from build123d import *

# Parameters (mm, degrees)
EXTRUDE_1_DEPTH              = 27
CUT_EXTRUDE_1_REACH          = 33.032
HOLE_WIZARD_M2_1_D           = 2.3
HOLE_WIZARD_M2_1_CBORE_D     = 3.8
HOLE_WIZARD_M2_1_CBORE_DEPTH = 0.5
PATTERN_LINEAR_1_COUNT       = 3
PATTERN_LINEAR_1_PITCH       = 10.5
MIRROR_1_COPY_1_D            = 2.3
MIRROR_1_COPY_1_CBORE_D      = 3.8
MIRROR_1_COPY_1_CBORE_DEPTH  = 0.5
MIRROR_1_COPY_2_D            = 2.3
MIRROR_1_COPY_2_CBORE_D      = 3.8
MIRROR_1_COPY_2_CBORE_DEPTH  = 0.5
CHAMFER_1_SIZE               = 1
MIRROR_3_COPY_1_D            = 2.3
MIRROR_3_COPY_1_CBORE_D      = 3.8
MIRROR_3_COPY_1_CBORE_DEPTH  = 0.5
MIRROR_3_COPY_2_D            = 2.3
MIRROR_3_COPY_2_CBORE_D      = 3.8
MIRROR_3_COPY_2_CBORE_DEPTH  = 0.5
MIRROR_3_COPY_3_D            = 2.3
MIRROR_3_COPY_3_CBORE_D      = 3.8
MIRROR_3_COPY_3_CBORE_DEPTH  = 0.5
MIRROR_3_COPY_4_D            = 2.3
MIRROR_3_COPY_4_CBORE_D      = 3.8
MIRROR_3_COPY_4_CBORE_DEPTH  = 0.5
MIRROR_3_COPY_5_D            = 2.3
MIRROR_3_COPY_5_CBORE_D      = 3.8
MIRROR_3_COPY_5_CBORE_DEPTH  = 0.5
CHAMFER_1_OF_MIRROR_3_SIZE   = 1
FILLET_1_R                   = 1.5
FILLET_2_R                   = 1
CHAMFER_2_SIZE               = 1.5
CUT_EXTRUDE_2_DEPTH          = 41.669398815


with BuildPart() as part:
    # ｽｹｯﾁ1 → ﾎﾞｽ - 押し出し1 (new, symmetric)
    with BuildSketch(Plane(origin=(0, 0, 0), x_dir=(0, 0, -1), z_dir=(1, 0, 0))):
        Polygon((-15, 0), (15, 0), (15, 5), (13, 5), (13, 2), (-13, 2), (-13, 5), (-15, 5), align=None)
    extrude(amount=EXTRUDE_1_DEPTH, both=True)

    # ｽｹｯﾁ2 → ｶｯﾄ - 押し出し1 (cut, up to next)
    with BuildSketch(Plane(origin=(0, 2, 0), x_dir=(1, 0, 0), z_dir=(0, 1, 0)), mode=Mode.PRIVATE) as cut_extrude_1_sk1:
        with BuildLine():
            Line((24, 6.75), (28, 6.75))
            Line((28, 6.75), (28, -6.75))
            Line((28, -6.75), (24, -6.75))
            ThreePointArc((24, -6.75), (17.25, 0), (24, 6.75))
        make_face()
    cut_extrude_1_tool1 = extrude(cut_extrude_1_sk1.sketch, amount=-CUT_EXTRUDE_1_REACH, mode=Mode.PRIVATE) & part.part
    cut_extrude_1 = cut_extrude_1_tool1.solids().sort_by_distance((23.22727, 2, 0))[0]
    add(cut_extrude_1, mode=Mode.SUBTRACT)

    # M2 丸平ねじ用座ぐり穴1 (through all)
    with Locations(Plane(origin=(0, 0, 0), x_dir=(-1, 0, 0), z_dir=(0, -1, 0))):
        with Locations((-24, -10.5)):
            hole_wizard_m2_1 = CounterBoreHole(HOLE_WIZARD_M2_1_D / 2, HOLE_WIZARD_M2_1_CBORE_D / 2, HOLE_WIZARD_M2_1_CBORE_DEPTH)

    # 直線ﾊﾟﾀｰﾝ1: M2 丸平ねじ用座ぐり穴1 ×3
    with Locations(*[(-i * PATTERN_LINEAR_1_PITCH, 0, 0) for i in range(1, PATTERN_LINEAR_1_COUNT)]):
        add(hole_wizard_m2_1, mode=Mode.SUBTRACT)

    # ﾐﾗｰ1: M2 丸平ねじ用座ぐり穴1 across plane
    add(hole_wizard_m2_1.mirror(Plane.XY), mode=Mode.SUBTRACT)

    # ﾐﾗｰ1 copy 1 (through all)
    with Locations(Plane(origin=(-10.5, 0, 0), x_dir=(-1, 0, 0), z_dir=(0, -1, 0))):
        with Locations((-24, 10.5)):
            CounterBoreHole(MIRROR_1_COPY_1_D / 2, MIRROR_1_COPY_1_CBORE_D / 2, MIRROR_1_COPY_1_CBORE_DEPTH)

    # ﾐﾗｰ1 copy 2 (through all)
    with Locations(Plane(origin=(-21, 0, 0), x_dir=(-1, 0, 0), z_dir=(0, -1, 0))):
        with Locations((-24, 10.5)):
            CounterBoreHole(MIRROR_1_COPY_2_D / 2, MIRROR_1_COPY_2_CBORE_D / 2, MIRROR_1_COPY_2_CBORE_DEPTH)

    # 面取り1
    chamfer_1_edges = [part.edges().sort_by_distance(p)[0] for p in [
        (25.5, 0, 6.75),
        (17.25, 0, 0),
        (25.5, 0, -6.75),
    ]]
    chamfer(chamfer_1_edges, length=CHAMFER_1_SIZE)

    # ﾐﾗｰ3: ｶｯﾄ - 押し出し1, M2 丸平ねじ用座ぐり穴1 across plane
    add(cut_extrude_1.mirror(Plane(origin=(0, 0, 0), x_dir=(0, 0, 1), z_dir=(1, 0, 0))), mode=Mode.SUBTRACT)
    add(hole_wizard_m2_1.mirror(Plane(origin=(0, 0, 0), x_dir=(0, 0, 1), z_dir=(1, 0, 0))), mode=Mode.SUBTRACT)

    # ﾐﾗｰ3 copy 1 (through all)
    with Locations(Plane(origin=(10.5, 0, 0), x_dir=(1, 0, 0), z_dir=(0, -1, 0))):
        with Locations((-24, 10.5)):
            CounterBoreHole(MIRROR_3_COPY_1_D / 2, MIRROR_3_COPY_1_CBORE_D / 2, MIRROR_3_COPY_1_CBORE_DEPTH)

    # ﾐﾗｰ3 copy 2 (through all)
    with Locations(Plane(origin=(21, 0, 0), x_dir=(1, 0, 0), z_dir=(0, -1, 0))):
        with Locations((-24, 10.5)):
            CounterBoreHole(MIRROR_3_COPY_2_D / 2, MIRROR_3_COPY_2_CBORE_D / 2, MIRROR_3_COPY_2_CBORE_DEPTH)

    # ﾐﾗｰ3 copy 3 (through all)
    with Locations(Plane.XZ):
        with Locations((-24, -10.5)):
            CounterBoreHole(MIRROR_3_COPY_3_D / 2, MIRROR_3_COPY_3_CBORE_D / 2, MIRROR_3_COPY_3_CBORE_DEPTH)

    # ﾐﾗｰ3 copy 4 (through all)
    with Locations(Plane(origin=(10.5, 0, 0), x_dir=(1, 0, 0), z_dir=(0, -1, 0))):
        with Locations((-24, -10.5)):
            CounterBoreHole(MIRROR_3_COPY_4_D / 2, MIRROR_3_COPY_4_CBORE_D / 2, MIRROR_3_COPY_4_CBORE_DEPTH)

    # ﾐﾗｰ3 copy 5 (through all)
    with Locations(Plane(origin=(21, 0, 0), x_dir=(1, 0, 0), z_dir=(0, -1, 0))):
        with Locations((-24, -10.5)):
            CounterBoreHole(MIRROR_3_COPY_5_D / 2, MIRROR_3_COPY_5_CBORE_D / 2, MIRROR_3_COPY_5_CBORE_DEPTH)

    # 面取り1 of ﾐﾗｰ3
    chamfer_1_of_mirror_3_edges = [part.edges().sort_by_distance(p)[0] for p in [
        (-25.5, 0, 6.75),
        (-17.25, 0, 0),
        (-25.5, 0, -6.75),
    ]]
    chamfer(chamfer_1_of_mirror_3_edges, length=CHAMFER_1_OF_MIRROR_3_SIZE)

    # ﾌｨﾚｯﾄ1
    fillet_1_edges = [part.edges().sort_by_distance(p)[0] for p in [
        (27, 2.5, -15),
        (-27, 2.5, 15),
        (27, 2.5, 15),
        (-27, 2.5, -15),
    ]]
    fillet(fillet_1_edges, radius=FILLET_1_R)

    # ﾌｨﾚｯﾄ2
    fillet_2_edges = [part.edges().sort_by_distance(p)[0] for p in [
        (27, 1.5, -6.75),
        (27, 1.5, 6.75),
        (-27, 1.5, -6.75),
        (-27, 1.5, 6.75),
    ]]
    fillet(fillet_2_edges, radius=FILLET_2_R)

    # 面取り2
    # the kernel refuses this chamfer: 1.5 mm, written as the material it takes off along each edge
    with BuildSketch(Plane(origin=(-29.357524482, 0, -15), x_dir=(0, -0.02749587661058654, 0.9996219169112965), z_dir=(1, 0, 0)), Plane(origin=(29.357524482, 0, 15), x_dir=(0, -0.027495876610586178, -0.9996219169112968), z_dir=(-1, 0, 0))) as chamfer_2_piece_1:
        Polygon((CHAMFER_2_SIZE * 0.999621916911, -CHAMFER_2_SIZE * 0.0274958766106), (-CHAMFER_2_SIZE * 0.0274958766106, -CHAMFER_2_SIZE * 0.999621916911), (0, 0), align=None)
    extrude(amount=58.715048964, mode=Mode.SUBTRACT)

    # ｽｹｯﾁ6 → ｶｯﾄ - 押し出し2 (cut, through all)
    with BuildSketch(Plane.XY.offset(15)):
        Polygon((27, 5), (16, 5), (27, 2), align=None)
        Polygon((11, 5), (-27, 5), (-27, 0), (0, 0), (0, 2), align=None)
    extrude(amount=-CUT_EXTRUDE_2_DEPTH, mode=Mode.SUBTRACT)


solid = part.part
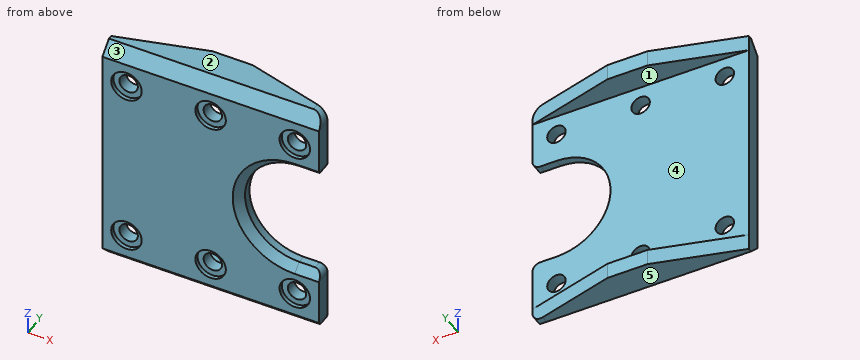
Could you check a few things on this model? Use its own coordinates, in mm. Face numbers are marked on the shaded views. A direction names the side the tool comes from. Give positions to 0.01 mm unless a question says otherwise; leave off trailing zeros. Order: outer loops, then holes, each group sorted by start corner. A loop starts at its lowest first (then second) coordinate and runs counter-clockwise, first axis right, second up.
1. I need wall thicknesses on L1, parallel to Z at x = 13.5, y = 1.55; L2, parallel to X at y = 1.2, z = 10.5; L3, parallel to X at y = 0.35, z = 10.5. Which ranges of each line are inside material? Lowest first, please.
2. Suppose I cut it at D-D (z = 0). List the corners of the cut face in (x, y) for me, plus the area to 3 significant figures.
3. Suppose I cut it at B-B (x = 13.5). List the corners of the cut face in (y, z) for me.
4. We'd pull the mould along Z, two halves only. Please class the marked faces 3, 4 and 5: pulls with the +Z half, pulls with the -Z half, needs draft (parallel to the pull), parting line crosses it, or undercut.
5. For the marked faces 1 and 2, which set-ups out of +Z, -Z, +X, -X, +Y, -Y let a thin tool reach every point of the face, with its end or its side?
6. Suppose I cut it at C-C (z = 10.5). List the corners of the cut face in (x, y) for me.
7. Will these pins go through, and if not, where does the flat tip stop? P1, Ø10, axis at x = 12.5, z = 10.5, coming from the -Y side; P2, Ø2, axis at x = 3, z = 10.5, coming from the -Y side; P3, Ø4.5, axis at x = 13.5, z = -10.5, coming from the +Y side; P4, Ø3, axis at x = 3, z = 10.5, coming from the -Y side.
8. Suppose I cut it at A-A (y = 3.05). List the corners of the cut face in (x, z) for me.
Solved:
1. L1: z = -15 to -11.65, -9.35 to 9.35, 11.65 to 15
1. L2: x = 0 to 1.85, 4.15 to 12.35, 14.65 to 22.85, 25.15 to 27
1. L3: x = 0 to 1.1, 4.9 to 11.6, 15.4 to 22.1, 25.9 to 27
2. outline: (0, 0) - (16.25, 0) - (17.25, 1) - (17.25, 2) - (0, 2) - close
2. area: 34.0 mm2
3. outline: (0, -13.5) - (1.5, -15) - (5, -15) - (5, -13) - (2, -13) - (2, -11.65) - (0.5, -11.65) - (0.5, -12.4) - (0, -12.4) - close; (0, -8.6) - (0.5, -8.6) - (0.5, -9.35) - (2, -9.35) - (2, 9.35) - (0.5, 9.35) - (0.5, 8.6) - (0, 8.6) - close; (0, 12.4) - (0.5, 12.4) - (0.5, 11.65) - (2, 11.65) - (2, 13) - (5, 13) - (5, 15) - (1.5, 15) - (0, 13.5) - close
4. face 3: pulls with the +Z half
4. face 4: undercut
4. face 5: pulls with the -Z half
5. face 1: +X, -X, +Y
5. face 2: +Z, +X, -X, +Y, -Y
6. outline: (0, 0) - (1.1, 0) - (1.1, 0.5) - (1.85, 0.5) - (1.85, 2) - (0, 2) - close; (4.15, 0.5) - (4.9, 0.5) - (4.9, 0) - (11.6, 0) - (11.6, 0.5) - (12.35, 0.5) - (12.35, 2) - (4.15, 2) - close; (14.65, 0.5) - (15.4, 0.5) - (15.4, 0) - (22.1, 0) - (22.1, 0.5) - (22.85, 0.5) - (22.85, 2) - (14.65, 2) - close; (25.15, 0.5) - (25.9, 0.5) - (25.9, 0) - (27, 0) - (27, 2) - (25.15, 2) - close
7. P1: stops at y = 0
7. P2: passes through
7. P3: stops at y = 2
7. P4: stops at y = 0.5
8. outline: (3.85, -15) - (23.15, -15) - (23.15, -13) - (3.85, -13) - close; (3.85, 13) - (23.15, 13) - (23.15, 15) - (3.85, 15) - close
